from build123d import *

# Parameters (mm, degrees)
SKETCH_1_W               = 105
SKETCH_1_H               = 135
SKETCH_1_R               = 1.5
EXTRUDE_1_DEPTH          = 1
SKETCH_3_W               = 113
SKETCH_3_H               = 143
SKETCH_3_W_2             = 107
SKETCH_3_H_2             = 137
EXTRUDE_2_DEPTH          = 8.5
SKETCH_3_3_W             = 113
SKETCH_3_3_H             = 143
EXTRUDE_3_DEPTH          = 8.5
CUT_EXTRUDE_1_DEPTH      = 6
CUT_EXTRUDE_1_DEPTH_BACK = 5
SKETCH_1_2_R             = 1.5
SKETCH_4_W               = 107
SKETCH_4_H               = 47.51
EXTRUDE_4_DEPTH          = 3.5
EXTRUDE_5_DEPTH          = 113


with BuildPart() as part:
    # Sketch 1 → Extrude 1 (new body)
    with BuildSketch(Plane.XY):
        with Locations((52.5, 67.5)):
            Rectangle(SKETCH_1_W, SKETCH_1_H)
        with Locations((3.61, 3.68)):
            Circle(SKETCH_1_R, mode=Mode.SUBTRACT)
        with Locations((101.26, 3.68)):
            Circle(SKETCH_1_R, mode=Mode.SUBTRACT)
        with Locations((3.61, 84.24)):
            Circle(SKETCH_1_R, mode=Mode.SUBTRACT)
        with Locations((101.26, 84.24)):
            Circle(SKETCH_1_R, mode=Mode.SUBTRACT)
    extrude(amount=EXTRUDE_1_DEPTH)



with BuildPart() as body_2:
    # Sketch 3 → Extrude 2 (new body)
    with BuildSketch(Plane.XY.offset(1)):
        with Locations((52.5, 67.5)):
            Rectangle(SKETCH_3_W, SKETCH_3_H)
        with Locations((52.5, 67.5)):
            Rectangle(SKETCH_3_W_2, SKETCH_3_H_2, mode=Mode.SUBTRACT)
    extrude(amount=EXTRUDE_2_DEPTH)


with BuildPart() as part_1:
    add(part.part)

    add(body_2.part)  # Extrude 3 merges body 2
    # Sketch 3_3 → Extrude 3 (add)
    with BuildSketch(Plane.XY.offset(1)):
        with Locations((52.5, 67.5)):
            Rectangle(SKETCH_3_3_W, SKETCH_3_3_H)
    extrude(amount=-EXTRUDE_3_DEPTH)

    # Sketch 1_2 → Cut-Extrude 1 (cut, two sides: drawn at the far end of the back side and taken through both)
    with BuildSketch(Plane.XY.offset(-CUT_EXTRUDE_1_DEPTH_BACK)):
        with Locations((3.61, 3.68)):
            Circle(SKETCH_1_2_R)
        with Locations((101.26, 3.68)):
            Circle(SKETCH_1_2_R)
        with Locations((3.61, 84.24)):
            Circle(SKETCH_1_2_R)
        with Locations((101.26, 84.24)):
            Circle(SKETCH_1_2_R)
    extrude(amount=CUT_EXTRUDE_1_DEPTH + CUT_EXTRUDE_1_DEPTH_BACK, mode=Mode.SUBTRACT)

    # Sketch 4 → Extrude 4 (add)
    with BuildSketch(Plane.XY.offset(1)):
        with Locations((52.5, 112.245)):
            Rectangle(SKETCH_4_W, SKETCH_4_H)
    extrude(amount=EXTRUDE_4_DEPTH)

    # Sketch 5 → Extrude 5 (add)
    with BuildSketch(Plane.ZY.offset(4)):
        Polygon((-7.5, 139), (-22.529905643, 139), (-7.5, -4), align=None)
    extrude(amount=-EXTRUDE_5_DEPTH)


solid = part_1.part
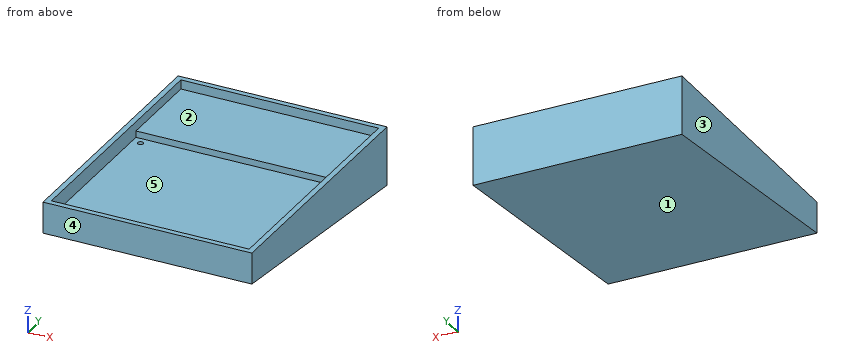
Design review of the part built by this model. Coordinates are the model's own, in mm. Face numbers are marked on the shaded views. A direction names the side the tool comes from. Round coordinates to 2 decimals unless told otherwise and drop trailing zeros. Loops run counter-clockwise (first coordinate to the right, second up) from the corner with the lowest first, then second, coordinate; pieces in that order, holes last. Notation, with made-up numbers: (32.25, 29) - (62.25, 29) arc R7 ccw to (62.25, 36) - close; hole circle Ø5 at (27.25, -40). An arc over 180 degrees is marked (long way). One line per question, with ' | ' between items.
1. We need section C-C, the plane x = 3.61. State the section outline as (y, z) points, and give its area (3 significant figures).
Results are:
outline: (-4, -7.5) - (139, -22.53) - (139, 9.5) - (136, 9.5) - (136, 4.5) - (88.49, 4.5) - (88.49, 1) - (85.74, 1) - (85.74, -5) - (82.74, -5) - (82.74, 1) - (5.18, 1) - (5.18, -5) - (2.18, -5) - (2.18, 1) - (-1, 1) - (-1, 9.5) - (-4, 9.5) - close | area: 2,470 mm²
2. For the marked faces 1 and 2, list the 3-axis set-ups (+Z, -Z, +X, -X, +Y, -Y) from which the entire face can be reached by the end or side of a thin tool; tool diameter is ignored.
Results are:
face 1: -Z, +X, -X, -Y | face 2: +Z
3. We need section A-A, the plane x = 93.5. State the section outline as (y, z) points, and give its area (3 significant figures).
Results are:
outline: (-4, -7.5) - (139, -22.53) - (139, 9.5) - (136, 9.5) - (136, 4.5) - (88.49, 4.5) - (88.49, 1) - (-1, 1) - (-1, 9.5) - (-4, 9.5) - close | area: 2,510 mm²
4. For L1, parallel to Y at x = 3.61, z = -2.9; L2, parallel to X at y = 84, z = -2; L3, parallel to Y at x = 101, z = 0, list the stretches that pass through material, from the lowest coordinate up. Write a range as [from, to].
Results are:
L1: y = [-4, 2.18], [5.18, 82.74], [85.74, 139] | L2: x = [-4, 2.13], [5.09, 99.78], [102.74, 109] | L3: y = [-4, 2.2], [5.16, 82.76], [85.72, 139]
5. Clearance check with flat-ended pins moving along their axes: P1, Ø8, axis at x = 38, y = 67, coming from the -Z side; P2, Ø2.5, axis at x = 3.61, y = 3.68, coming from the +Z side; P3, Ø2, axis at x = 95, y = 18.5, coming from the -Z side. State where each tip first meets the part, or that it passes through.
Results are:
P1: stops at z = -15.38 | P2: stops at z = -5 | P3: stops at z = -9.97
6. We need section B-B, the plane y = 3.68. State the section outline as (x, z) points.
Results are:
outline: (-4, -8.31) - (109, -8.31) - (109, 9.5) - (106, 9.5) - (106, 1) - (102.76, 1) - (102.76, -5) - (99.76, -5) - (99.76, 1) - (5.11, 1) - (5.11, -5) - (2.11, -5) - (2.11, 1) - (-1, 1) - (-1, 9.5) - (-4, 9.5) - close
7. We need section D-D, the plane z = -18. State the section outline as (x, y) points, and give its area (3 significant figures).
Results are:
outline: (-4, 95.9) - (109, 95.9) - (109, 139) - (-4, 139) - close | area: 4,870 mm²
8. Draft analysis for pull direction Y (two halves, no side actions). For the marked faces 3, 4 and 5, state which applies: released by +Y, released by -Y, zero draft, split by the parting line, or undercut.
Results are:
face 3: zero draft | face 4: released by -Y | face 5: undercut
